Could you check a few things on this model? Use its own coordinates, in mm. Face numbers are marked on the shaded views. A direction names the side the tool comes from. Give positions to 0.01 mm unless a question says otherwise; leave off trailing zeros. Loops run counter-clockwise (first coordinate to the right, second up) from the corner with the lowest first, then second, coordinate; pieces in that order, holes last. Notation, with made-up numbers: (0.25, 57.5) -> (40.25, 57.5) arc R31 ccw to (40.25, 93.5) -> close; hole circle Ø7 at (26, 86). An arc over 180 degrees is marked (long way). Write item = value, one per line. Start each with the question number.
1) I want a section at A-A (z = -25). List the corners of the cut face in (x, y) for me, and give its area (3 significant figures).
2) I want a section at D-D (z = -19.75). List the corners of the cut face in (x, y) for me.
3) If we mould it in two halves opening along Z, with no side actions, what happens to the marked faces 1, 2 and 3? For each: +Z half, -Z half, draft (parallel to the pull), parting line (faces both ways), or undercut.
4) On a 3-axis mill with a long thin cutter (end or side, diameter ignored), from which of +Z, -Z, +X, -X, +Y, -Y can I reach the whole of each face in a straight line? I mean the marked faces 4, 5 and 6. Say none if no direction works.
5) I want a section at C-C (x = 25.5). List the corners of the cut face in (y, z) for me.
6) I want a section at B-B (y = 59.75). List the corners of the cut face in (x, z) for me.
7) I'm going to push flat-ended pins straight in: pin 1 Ø5 at (x, z) = (16.5, -27) entering from -Y; pin 2 Ø3 at (x, z) = (5, -25) entering from +Y. Where does each tip first touch, or does it pass through?
8) I need wall thicknesses on probe 1 along X at (y, z) = (59.6, -25); probe 2 along Z at (x, y) = (5, 57.9); probe 3 along X at (y, z) = (55.75, -30). Which ranges of each line are inside material? Lowest first, please. Write a range as from..to.
from build123d import *

# Parameters (mm, degrees)
SKETCH_1_W           = 30
SKETCH_1_H           = 61.5
EXTRUDE_1_DEPTH      = 5
SKETCH_2_R           = 1.75
SKETCH_2_W           = 21
SKETCH_2_H           = 41
CUT_EXTRUDE_1_DEPTH  = 6
SKETCH_3_W           = 30
SKETCH_3_H           = 40
EXTRUDE_2_DEPTH      = 5
SKETCH_4_R           = 1.75
CUT_EXTRUDE_2_DEPTH  = 62.5
SKETCH_5_W           = 10
SKETCH_5_H           = 12
EXTRUDE_3_DEPTH      = 2.3
SKETCH_6_W           = 30
SKETCH_6_H           = 12
EXTRUDE_4_DEPTH      = 4
EXTRUDE_5_DEPTH      = 4.5
FILLET_1_R           = 5
SKETCH_8_W           = 21
SKETCH_8_H           = 6
CUT_EXTRUDE_3_DEPTH  = 10
SKETCH_9_OUTSIDE_W   = 63.988
SKETCH_9_OUTSIDE_H   = 84.488
SKETCH_9_OUTSIDE_W_2 = 12
SKETCH_9_OUTSIDE_H_2 = 7.3
CUT_EXTRUDE_4_DEPTH  = 31


with BuildPart() as part:
    # ｽｹｯﾁ1 → ﾎﾞｽ - 押し出し1 (new body)
    with BuildSketch(Plane.XY):
        with Locations((15, 30.75)):
            Rectangle(SKETCH_1_W, SKETCH_1_H)
    extrude(amount=EXTRUDE_1_DEPTH)

    # ｽｹｯﾁ2 → ｶｯﾄ - 押し出し1 (cut, through all)
    with BuildSketch(Plane.XY.offset(5)):
        with Locations((10, 3.5)):
            Circle(SKETCH_2_R)
        with Locations((20, 3.5)):
            Circle(SKETCH_2_R)
        with Locations((10, 53)):
            Circle(SKETCH_2_R)
        with Locations((20, 53)):
            Circle(SKETCH_2_R)
        with Locations((15, 28.2)):
            Rectangle(SKETCH_2_W, SKETCH_2_H)
    extrude(amount=-CUT_EXTRUDE_1_DEPTH, mode=Mode.SUBTRACT)

    # ｽｹｯﾁ3 → ﾎﾞｽ - 押し出し2 (add)
    with BuildSketch(Plane(origin=(0, 61.5, 0), x_dir=(1, 0, 0), z_dir=(0, 1, 0))):
        with Locations((15, 20)):
            Rectangle(SKETCH_3_W, SKETCH_3_H)
    extrude(amount=-EXTRUDE_2_DEPTH)

    # ｽｹｯﾁ4 → ｶｯﾄ - 押し出し2 (cut, through all)
    with BuildSketch(Plane(origin=(0, 61.5, 0), x_dir=(1, 0, 0), z_dir=(0, 1, 0))):
        with Locations((5, 25)):
            Circle(SKETCH_4_R)
        with Locations((25, 25)):
            Circle(SKETCH_4_R)
    extrude(amount=-CUT_EXTRUDE_2_DEPTH, mode=Mode.SUBTRACT)

    # ｽｹｯﾁ5 → ﾎﾞｽ - 押し出し3 (add)
    with BuildSketch(Plane.XZ.offset(-56.5)):
        with Locations((5, -25)):
            Rectangle(SKETCH_5_W, SKETCH_5_H)
        Polygon((5, -28.6), (8.117691454, -26.8), (8.117691454, -23.2), (5, -21.4), (1.882308546, -23.2), (1.882308546, -26.8), align=None, mode=Mode.SUBTRACT)
        with Locations((25, -25)):
            Rectangle(SKETCH_5_W, SKETCH_5_H)
        Polygon((28.117691454, -26.8), (25, -28.6), (21.882308546, -26.8), (21.882308546, -23.2), (25, -21.4), (28.117691454, -23.2), align=None, mode=Mode.SUBTRACT)
    extrude(amount=EXTRUDE_3_DEPTH)

    # ｽｹｯﾁ6 → ﾎﾞｽ - 押し出し4 (add)
    with BuildSketch(Plane(origin=(0, 61.5, 0), x_dir=(1, 0, 0), z_dir=(0, 1, 0))):
        with Locations((15, 1)):
            Rectangle(SKETCH_6_W, SKETCH_6_H)
    extrude(amount=EXTRUDE_4_DEPTH)

    # ｽｹｯﾁ7 → ﾎﾞｽ - 押し出し5 (add)
    with BuildSketch(Plane(origin=(30, 0, 0), x_dir=(0, 0, -1), z_dir=(1, 0, 0))):
        Polygon((40, 56.5), (40, 39.5), (0, 9.822580645), (0, 21.5), (31, 44.5), (31, 56.5), align=None)
    extrude_5 = extrude(amount=-EXTRUDE_5_DEPTH)

    # ﾐﾗｰ1: ﾎﾞｽ - 押し出し5 across plane
    add(extrude_5.mirror(Plane.ZY.offset(-15)))

    # ﾌｨﾚｯﾄ1
    fillet_1_edges = [part.edges().sort_by_distance(p)[0] for p in [
        (30, 0, 2.5),
        (0, 0, 2.5),
    ]]
    fillet(fillet_1_edges, radius=FILLET_1_R)

    # ｽｹｯﾁ8 → ｶｯﾄ - 押し出し3 (cut, through all)
    with BuildSketch(Plane.XZ.offset(-56.5)):
        with Locations((15, -37)):
            Rectangle(SKETCH_8_W, SKETCH_8_H)
    extrude(amount=-CUT_EXTRUDE_3_DEPTH, mode=Mode.SUBTRACT)

    # ｽｹｯﾁ9 outside → ｶｯﾄ - 押し出し4 (cut, through all)
    with BuildSketch(Plane.ZY):
        with Locations((-17.5, 32.75)):
            Rectangle(SKETCH_9_OUTSIDE_W, SKETCH_9_OUTSIDE_H)
        with Locations((-25, 57.85)):
            Rectangle(SKETCH_9_OUTSIDE_W_2, SKETCH_9_OUTSIDE_H_2, mode=Mode.SUBTRACT)
    extrude(amount=-CUT_EXTRUDE_4_DEPTH, mode=Mode.SUBTRACT)


solid = part.part
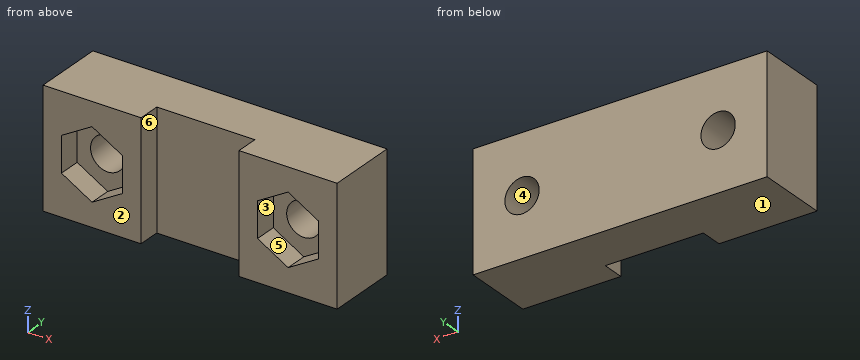
Answer list:
q1.outline = (0, 54.2) -> (1.88, 54.2) -> (1.88, 56.5) -> (3.25, 56.5) -> (3.25, 61.5) -> (0, 61.5) -> close; (6.75, 56.5) -> (8.12, 56.5) -> (8.12, 54.2) -> (10, 54.2) -> (10, 56.5) -> (20, 56.5) -> (20, 54.2) -> (21.88, 54.2) -> (21.88, 56.5) -> (23.25, 56.5) -> (23.25, 61.5) -> (6.75, 61.5) -> close; (26.75, 56.5) -> (28.12, 56.5) -> (28.12, 54.2) -> (30, 54.2) -> (30, 61.5) -> (26.75, 61.5) -> close
q1.area = 132 mm^2
q2.outline = (0, 54.2) -> (10, 54.2) -> (10, 56.5) -> (20, 56.5) -> (20, 54.2) -> (30, 54.2) -> (30, 61.5) -> (0, 61.5) -> close
q3.face_1 = -Z half
q3.face_2 = draft
q3.face_3 = undercut
q4.face_4 = +Y, -Y
q4.face_5 = -Y
q4.face_6 = +Z, -Z, -Y
q5.outline = (54.2, -31) -> (61.5, -31) -> (61.5, -26.68) -> (56.5, -26.68) -> (56.5, -28.31) -> (54.2, -28.31) -> close; (54.2, -21.69) -> (56.5, -21.69) -> (56.5, -23.32) -> (61.5, -23.32) -> (61.5, -19) -> (54.2, -19) -> close
q6.outline = (0, -31) -> (30, -31) -> (30, -19) -> (0, -19) -> close; hole circle Ø3.5 at (5, -25); hole circle Ø3.5 at (25, -25)
q7.pin_1 = 56.5
q7.pin_2 = through
q8.probe_1 = 0..3.25, 6.75..23.25, 26.75..30
q8.probe_2 = -31..-26.75, -23.25..-19
q8.probe_3 = 0..10, 20..30
